Autodesk Inventor part; units mm, degrees
ref_plane "YZ Plane" through (0, 0, 0) normal (1, 0, 0) x (0, 1, 0)
ref_plane "XZ Plane" through (0, 0, 0) normal (0, 1, 0) x (-1, 0, 0)
ref_plane "XY Plane" through (0, 0, 0) normal (0, 0, 1) x (1, 0, 0)
sketch "Sketch1" plane through (0, 0, 0) normal (0, 0, 1) x (1, 0, 0)
  line L0 (0, 0) -> (1420, 0)
  line L1 (1420, 0) -> (1420, 695)
  line L2 (1420, 695) -> (0, 695)
  line L3 (0, 695) -> (0, 0)
  dimension "d0" = 695
  dimension "d1" = 1420
extrude "Extrusion1" add sketch "Sketch1" along normal blind 670
sketch "Sketch2" plane through (1420, 0, 0) normal (1, 0, 0) x (0, 0, -1)
  line L0 (-630, 0) -> (-40, 0)
  line L1 (-40, 0) -> (-40, 420)
  line L2 (-40, 420) -> (-630, 420)
  line L3 (-630, 420) -> (-630, 0)
  line L4 (-670, 695) -> (-670, 0)
  line L5 (0, 0) -> (0, 695)
  line L6 (0, 0) -> (-670, 0)
  dimension "d4" = 420
  dimension "d5" = 40
  dimension "d6" = 40
extrude "Extrusion2" cut sketch "Sketch2" against normal blind 2000
sketch "Sketch3" plane through (1420, 0, 0) normal (1, 0, 0) x (0, 0, -1)
  line L0 (-630, 460) -> (-40, 460)
  line L1 (-40, 460) -> (-40, 655)
  line L2 (-40, 655) -> (-630, 655)
  line L3 (-630, 655) -> (-630, 460)
  line L4 (0, 695) -> (-670, 695)
  line L5 (-670, 695) -> (-670, 0)
  line L6 (-630, 420) -> (-40, 420)
  line L7 (0, 0) -> (0, 695)
  dimension "d9" = 40
  dimension "d10" = 40
  dimension "d11" = 40
  dimension "d12" = 40
extrude "Extrusion3" cut sketch "Sketch3" against normal blind 2000
sketch "Sketch4" plane through (0, 0, 670) normal (0, 0, 1) x (1, 0, 0)
  line L0 (40, 0) -> (1380, 0)
  line L1 (1380, 0) -> (1380, 655)
  line L2 (1380, 655) -> (40, 655)
  line L3 (40, 655) -> (40, 0)
  line L4 (0, 0) -> (1420, 0)
  line L5 (0, 420) -> (0, 0)
  line L6 (1420, 0) -> (1420, 695)
  line L7 (1420, 695) -> (0, 695)
  dimension "d15" = 40
  dimension "d16" = 40
  dimension "d17" = 40
extrude "Extrusion4" cut sketch "Sketch4" against normal blind 1000
properties part number "bottomtable"
CAD build for the part. Positions are in the model's coordinates, mm. A direction names the side the tool comes from. Coordinates: 2 decimals unless noted, no trailing zeros. Order: outer loops, then holes, each group sorted by start corner. A loop starts at its lowest first (then second) coordinate and runs counter-clockwise, first axis right, second up. Notation, with made-up numbers: M -12.75,76.5 L 10.25,76.5 A38 cw 10.25,114.5 Z; hole C -32.5,12.5 d11. An arc over 180 degrees is marked long. Write each question's results on one line, items separated by ' | '. Start each with the question number.
Q1. Drill centre lines: probe 1 along X at (y, z) = (441, 307); probe 2 along Y at (x, z) = (1031.5, 64). Where is each one in solid material? Low to high. Write a range as from..to.
Q2. Which spindle directions (+Z, -Z, +X, -X, +Y, -Y) get a long thin tool onto all of the face, cutting with end or side? Do faces 4 (the flat face through (1400, 213, 630)), 5 (the flat face through (1400, 559, 630)), 6 (the flat face through (0, 426, 333)). Say none if no direction does.
Q3. Cut at B-B (z = 581.5). List the corners of the cut face in (x, y), then the cut area to 3 significant figures.
Q4. Cut at A-A (y = 234.5). List the corners of the cut face in (x, z), then the cut area to 3 significant figures.
Q5. Cut at C-C (x = 1058). List the corners of the cut face in (y, z), then the cut area to 3 significant figures.
Q6. Pull direction Y, two halves, no side cores. Call faces 1 (the flat face through (20, 556, 40)), 2 (the flat face through (1400, 0, 650)), 3 (the flat face through (654, 658, 0)): +Y half, -Y half, draft (parallel to the pull), parting line (faces both ways), or undercut.
Q7. Flat gauge pins, fed straight in: P1, Ø20, axis at x = 1405.5, y = 189.5, coming from the -Z side; P2, Ø5, axis at x = 589, z = 149, coming from the -Y side; P3, Ø12, axis at x = 1410, z = 195.5, coming from the -Y side. Where does each tip first touch, or does it go through?
Found:
1) probe 1: 0..40, 1380..1420 | probe 2: 655..695
2) face 4: +X, -X, -Y | face 5: +X, -X | face 6: +Z, -Z, -X, +Y, -Y
3) outline: M 0,420 L 40,420 L 40,460 L 0,460 Z; M 0,655 L 1420,655 L 1420,695 L 0,695 Z; M 1380,420 L 1420,420 L 1420,460 L 1380,460 Z | area: 60,000 mm²
4) outline: M 0,0 L 40,0 L 40,40 L 0,40 Z; M 0,630 L 40,630 L 40,670 L 0,670 Z; M 1380,0 L 1420,0 L 1420,40 L 1380,40 Z; M 1380,630 L 1420,630 L 1420,670 L 1380,670 Z | area: 6,400 mm²
5) outline: M 655,0 L 695,0 L 695,670 L 655,670 Z | area: 26,800 mm²
6) face 1: undercut | face 2: -Y half | face 3: draft
7) P1: z = 0 | P2: y = 655 | P3: y = 420
